Work out the finished part from the listing and answer in its coordinate system (mm). Round coordinates to 2 decimals unless told otherwise and drop trailing zeros. Loops run counter-clockwise (first coordinate to the right, second up) from the corner with the lowest first, then second, coordinate; pieces in that order, holes last. Notation, with made-up numbers: (17.25, -21) -> (65.25, -21) arc R28 ccw to (65.25, 15) -> close; hole circle Ø1 at (45.5, 49.5). An arc over 180 degrees is marked (long way). Use one line per item in the form item = value.
```python
from build123d import *

# Parameters (mm, degrees)
SKETCH1_R           = 1.375
SKETCH1_R_2         = 10
BOSS_EXTRUDE1_DEPTH = 2.7


with BuildPart() as part:
    # Sketch1 → Boss-Extrude1 (new body)
    with BuildSketch(Plane.XY):
        Polygon((30, -47.3), (30, 50), (30, 60), (-30, 60), (-30, 50), (-30, -47.3), (-18, -47.3), (-18, -50), (-6, -50), (-6, -47.3), (6, -47.3), (6, -50), (18, -50), (18, -47.3), align=None)
        with Locations((-24.5, 45)):
            Circle(SKETCH1_R, mode=Mode.SUBTRACT)
        with Locations((24.5, 45)):
            Circle(SKETCH1_R, mode=Mode.SUBTRACT)
        with Locations((-24.5, -13)):
            Circle(SKETCH1_R, mode=Mode.SUBTRACT)
        with Locations((24.5, -13)):
            Circle(SKETCH1_R, mode=Mode.SUBTRACT)
        with Locations((0, 16)):
            Circle(SKETCH1_R_2, mode=Mode.SUBTRACT)
        with Locations((0, 41)):
            Circle(SKETCH1_R_2, mode=Mode.SUBTRACT)
        with Locations((0, -9)):
            Circle(SKETCH1_R_2, mode=Mode.SUBTRACT)
    extrude(amount=BOSS_EXTRUDE1_DEPTH)


solid = part.part
```
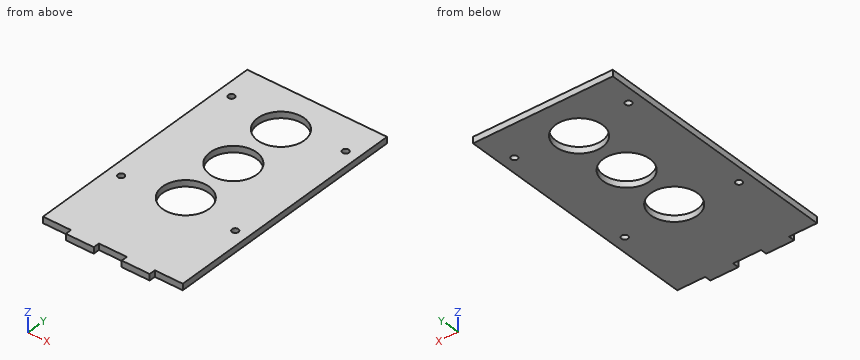
(1) Find section B-B, the plane x = 0. Write down the section's boundary in (y, z), then the cut area to 3 significant figures.
Completed:
outline = (-47.3, 0) -> (-19, 0) -> (-19, 2.7) -> (-47.3, 2.7) -> close; (1, 0) -> (6, 0) -> (6, 2.7) -> (1, 2.7) -> close; (26, 0) -> (31, 0) -> (31, 2.7) -> (26, 2.7) -> close; (51, 0) -> (60, 0) -> (60, 2.7) -> (51, 2.7) -> close
area = 128 mm2
(2) Find section D-D, the plane z = 1.9. Write down the section's boundary in (x, y) (3 decimals).
Completed:
outline = (-30, -47.3) -> (-18, -47.3) -> (-18, -50) -> (-6, -50) -> (-6, -47.3) -> (6, -47.3) -> (6, -50) -> (18, -50) -> (18, -47.3) -> (30, -47.3) -> (30, 60) -> (-30, 60) -> close; hole circle Ø2.75 at (-24.5, -13); hole circle Ø2.75 at (-24.5, 45); hole circle Ø20 at (0, -9); hole circle Ø20 at (0, 16); hole circle Ø20 at (0, 41); hole circle Ø2.75 at (24.5, -13); hole circle Ø2.75 at (24.5, 45)
(3) Given P1, Ø1, axis at x = -3, z = 1, coming from the -Y side; P2, Ø1.4, axis at y = -49.5, z = 2, coming from the -X side, each flat-ended and moving along its own axis, determine where each tip first touches the part or whether it passes through.
Completed:
P1 = -47.3
P2 = -18
(4) Find section C-C, the plane x = 24.5. Write down the section's boundary in (y, z) (3 decimals).
Completed:
outline = (-47.3, 0) -> (-14.375, 0) -> (-14.375, 2.7) -> (-47.3, 2.7) -> close; (-11.625, 0) -> (43.625, 0) -> (43.625, 2.7) -> (-11.625, 2.7) -> close; (46.375, 0) -> (60, 0) -> (60, 2.7) -> (46.375, 2.7) -> close
(5) Consider L1, parallel to Y at x = -24.5, z = 2 (3 decimals); L2, parallel to Y at x = 0.5, z = 1.8; L3, parallel to Y at x = 4.5, z = 2.45. Determine where each line is inside the solid, lowest interval first.
Completed:
L1 = -47.3 to -14.375, -11.625 to 43.625, 46.375 to 60
L2 = -47.3 to -18.99, 0.99 to 6.01, 25.99 to 31.01, 50.99 to 60
L3 = -47.3 to -17.93, -0.07 to 7.07, 24.93 to 32.07, 49.93 to 60
(6) Find section A-A, the plane y = 41. Write down the section's boundary in (x, z).
Completed:
outline = (-30, 0) -> (-10, 0) -> (-10, 2.7) -> (-30, 2.7) -> close; (10, 0) -> (30, 0) -> (30, 2.7) -> (10, 2.7) -> close
